The listing builds one solid part. Answer for the finished solid, in the listing's coordinates (mm). Face numbers are marked on the shaded views. A direction names the side the tool comes from. Give positions to 0.01 mm unless a question says otherwise; leave off trailing zeros. Loops run counter-clockwise (first coordinate to the right, second up) from the corner with the lowest first, then second, coordinate; pieces in that order, holes last. Notation, with made-up numbers: (64.5, 81.5) - (122.5, 81.5) arc R20 ccw to (122.5, 115.5) - close; hole circle Ø1 at (23, 12). An arc over 180 degrees is marked (long way). Write each question's results on one line, items separated by ' | '.
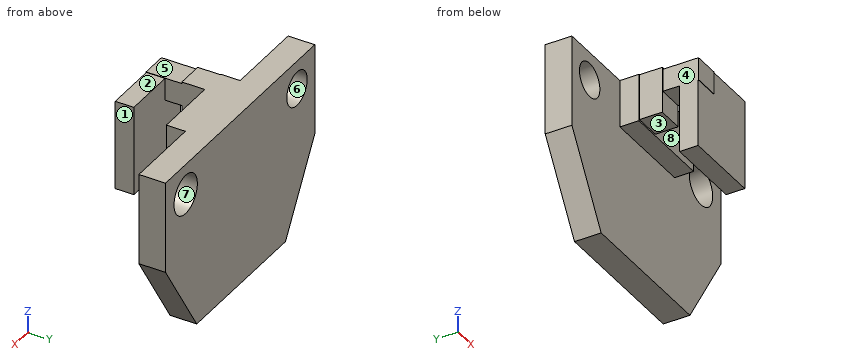
from build123d import *

# Parameters (mm, degrees)
F0_W      = 83.9228034019
F0_H      = 30.6277740747
F1_DEPTH  = 8.89
F2_W      = 30.7626985013
F2_H      = 15.9210450947
F3_DEPTH  = 15.24
F4_W      = 8.9049930684
F4_H      = 15.3813483194
F5_DEPTH  = 22.86
F6_W      = 8.6351442151
F6_H      = 7.55575113
F7_DEPTH  = 34.798
F8_W      = 26.175278239
F8_H      = 6.2065087259
F9_DEPTH  = 29.972
F10_R     = 5.7243436082
F10_R_2   = 6.565694646
F11_DEPTH = 25.4


with BuildPart() as f1:
    # F0 (on Front) → F1 (new body)
    with BuildSketch(Plane.XZ):
        with Locations((-0.9444691241, 15.3138870373)):
            Rectangle(F0_W, F0_H)
        Polygon((41.0169325769, 0), (-42.9058708251, 0), (-26.445126161, -27.6594422758), (23.4767943621, -27.6594422758), align=None)
    extrude(amount=F1_DEPTH)

    # F2 (on Front) → F3 (join)
    with BuildSketch(Plane.XZ):
        with Locations((-0.5396958441, 22.6672515273)):
            Rectangle(F2_W, F2_H)
    extrude(amount=F3_DEPTH)

    # F4 (on Front) → F5 (join)
    with BuildSketch(Plane.XZ):
        with Locations((-11.1987015698, 22.937099915)):
            Rectangle(F4_W, F4_H)
    extrude(amount=F5_DEPTH)

    # F6 (on Front) → F7 (join)
    with BuildSketch(Plane.XZ):
        with Locations((-11.0637771431, 26.3102026656)):
            Rectangle(F6_W, F6_H)
    extrude(amount=F7_DEPTH)

    # F8 (on Top) → F9 (join)
    with BuildSketch(Plane.XY):
        with Locations((-2.2937101312, -31.5722431988)):
            Rectangle(F8_W, F8_H)
    extrude(amount=F9_DEPTH)

    # F10 (on Front) → F11 (cut)
    with BuildSketch(Plane.XZ):
        with Locations((-32.9214856029, 21.1830865592)):
            Circle(F10_R)
        with Locations((29.6833030879, 20.3735418618)):
            Circle(F10_R_2)
    extrude(amount=F11_DEPTH, mode=Mode.SUBTRACT)


solid = f1.part
Item 1: A cutting plane is placed at C-C, the plane x = -11. Determine the outline of the cut face in (y, z), plus the area to 3 significant figures.
Values found:
outline: (-34.8, 22.53) - (-34.68, 22.53) - (-34.68, 0) - (-28.47, 0) - (-28.47, 22.53) - (-22.86, 22.53) - (-22.86, 15.25) - (-15.24, 15.25) - (-15.24, 14.71) - (-8.89, 14.71) - (-8.89, -27.66) - (0, -27.66) - (0, 30.63) - (-22.86, 30.63) - (-22.86, 30.09) - (-34.8, 30.09) - close | area: 967 mm²
Item 2: Flat-ended cylindrical pins translate along their axes: P1, Ø3, axis at x = -5, y = -13.5, coming from the -Z side; P2, Ø5, axis at y = -12, z = 24.5, coming from the -X side; P3, Ø13, axis at x = -3, z = 8, coming from the -Y side; P4, Ø12, axis at x = -22, y = -15, coming from the -Z side. Find the tip coordinate at first contact, or state that the pin passes through.
Values found:
P1: stops at z = 14.71 | P2: stops at x = -15.92 | P3: stops at y = -34.68 | P4: passes through
Item 3: For a pull along Z with two mould halves and no side action, classify the marked faces 5, 6, 7 and 8 as released by +Z, released by -Z, zero draft, split by the parting line, or undercut.
Values found:
face 5: released by +Z | face 6: undercut | face 7: undercut | face 8: zero draft
Item 4: Find the intervals of material crossed by line 1 along Y through (x, z) = (4, 11); line 2 along Y through (x, z) = (1, -2); line 3 along X through (y, z) = (-31.5, 21), in increasing order. Write a range as [from, to].
Values found:
line 1: y = [-34.68, -28.47], [-8.89, 0] | line 2: y = [-8.89, 0] | line 3: x = [-15.38, 10.79]
Item 5: A cutting plane is placed at B-B, the plane z = 8. Determine the outline of the cut face in (x, y).
Values found:
outline: (-42.91, -8.89) - (41.02, -8.89) - (41.02, 0) - (-42.91, 0) - close; (-15.38, -34.68) - (10.79, -34.68) - (10.79, -28.47) - (-15.38, -28.47) - close
Item 6: A cutting plane is placed at D-D, the plane y = -5. Determine the outline of the cut face in (x, z).
Values found:
outline: (-42.91, 0) - (-26.45, -27.66) - (23.48, -27.66) - (41.02, 0) - (41.02, 30.63) - (-42.91, 30.63) - close; hole circle Ø11.45 at (-32.92, 21.18); hole circle Ø13.13 at (29.68, 20.37)
Item 7: For the marked faces 1, 2, 3 and 4, determine the directions among +Z, -Z, +X, -X, +Y, -Y from which every point of the face is accessible in a straight line to the end or side of a thin tool.
Values found:
face 1: +Z, -Z, +X, -Y | face 2: +Z, +X, -Y | face 3: -Z, +X, -X | face 4: +Z, -Z, -X, -Y
Item 8: A cutting plane is placed at A-A, the plane x = 5.5. Determine the outline of the cut face in (y, z), plus the area to 3 significant figures.
Values found:
outline: (-34.68, 0) - (-28.47, 0) - (-28.47, 29.97) - (-34.68, 29.97) - close; (-15.24, 14.71) - (-8.89, 14.71) - (-8.89, -27.66) - (0, -27.66) - (0, 30.63) - (-15.24, 30.63) - close | area: 805 mm²
